```python
from build123d import *

# Parameters (mm, degrees)
SKETCH1_W                        = 6.5
SKETCH1_H                        = 60
BOSS_EXTRUDE1_DEPTH              = 6.25
CUT_EXTRUDE3_DEPTH               = 61.673820549
LPATTERN1_COUNT                  = 12
LPATTERN1_PITCH                  = 2
CBORE_FOR_M1_6_SHCS1_D           = 2.8
CBORE_FOR_M1_6_SHCS1_CBORE_D     = 5.6
CBORE_FOR_M1_6_SHCS1_CBORE_DEPTH = 1.5
SKETCH6_W                        = 1
SKETCH6_H                        = 40
CUT_EXTRUDE2_DEPTH               = 61.673820549


with BuildPart() as part:
    # Sketch1 → Boss-Extrude1 (new body)
    with BuildSketch(Plane(origin=(0, 0, 0), x_dir=(1, 0, 0), z_dir=(0, 1, 0))):
        with Locations((3.25, 30)):
            Rectangle(SKETCH1_W, SKETCH1_H)
    extrude(amount=BOSS_EXTRUDE1_DEPTH)

    # Sketch9 → Cut-Extrude3 (cut, through all)
    with BuildSketch(Plane.ZY):
        with BuildLine():
            Line((-19, 6.25), (-15, 6.25))
            Line((-15, 6.25), (-15, 5.62))
            Line((-15, 5.62), (-15.259824575, 5.62))
            ThreePointArc((-15.259824575, 5.62), (-15.358731646, 5.582771412), (-15.408543109, 5.489565217))
            ThreePointArc((-15.408543109, 5.489565217), (-15.442388286, 5.331937846), (-15.501123596, 5.181797753))
            ThreePointArc((-15.501123596, 5.181797753), (-16, 4.87), (-16.498876404, 5.181797753))
            ThreePointArc((-16.498876404, 5.181797753), (-16.557611714, 5.331937846), (-16.591456891, 5.489565217))
            ThreePointArc((-16.591456891, 5.489565217), (-16.641268354, 5.582771412), (-16.740175425, 5.62))
            Line((-16.740175425, 5.62), (-17.259824575, 5.62))
            ThreePointArc((-17.259824575, 5.62), (-17.358731646, 5.582771412), (-17.408543109, 5.489565217))
            ThreePointArc((-17.408543109, 5.489565217), (-17.442388286, 5.331937846), (-17.501123596, 5.181797753))
            ThreePointArc((-17.501123596, 5.181797753), (-18, 4.87), (-18.498876404, 5.181797753))
            ThreePointArc((-18.498876404, 5.181797753), (-18.557611714, 5.331937846), (-18.591456891, 5.489565217))
            ThreePointArc((-18.591456891, 5.489565217), (-18.641268354, 5.582771412), (-18.740175425, 5.62))
            Line((-18.740175425, 5.62), (-19, 5.62))
            Line((-19, 5.62), (-19, 6.25))
        make_face()
    cut_extrude3 = extrude(amount=-CUT_EXTRUDE3_DEPTH, mode=Mode.SUBTRACT)

    # LPattern1: Cut-Extrude3 ×12
    with Locations(*[(0, 0, -i * LPATTERN1_PITCH) for i in range(1, LPATTERN1_COUNT)]):
        add(cut_extrude3, mode=Mode.SUBTRACT)

    # CBORE for M1.6 SHCS1 (through all)
    with Locations(Plane(origin=(0, 6.25, 0), x_dir=(1, 0, 0), z_dir=(0, 1, 0))):
        with Locations((3.25, 55), (3.25, 5)):
            CounterBoreHole(CBORE_FOR_M1_6_SHCS1_D / 2, CBORE_FOR_M1_6_SHCS1_CBORE_D / 2, CBORE_FOR_M1_6_SHCS1_CBORE_DEPTH)

    # Sketch6 → Cut-Extrude2 (cut, through all)
    with BuildSketch(Plane(origin=(0, 6.25, 0), x_dir=(1, 0, 0), z_dir=(0, 1, 0))):
        with Locations((6, 20)):
            Rectangle(SKETCH6_W, SKETCH6_H)
        with Locations((0.5, 20)):
            Rectangle(SKETCH6_W, SKETCH6_H)
    extrude(amount=-CUT_EXTRUDE2_DEPTH, mode=Mode.SUBTRACT)


solid = part.part
```
Build history of the part. All positions in model axes, mm. A direction names the side the tool comes from. Round coordinates to 2 decimals unless told otherwise and drop trailing zeros. Write each loop counter-clockwise with the first axis right and the second up, starting at its lowest first coordinate (ties: lowest second). Pieces come first, ordered by that corner, then holes. Notation, with made-up numbers: (77.5, 75) -> (102.5, 75) arc R30 ccw to (102.5, 100) -> close; hole circle Ø9 at (-23.75, 24). An arc over 180 degrees is marked (long way). Put each result on its own line as item: value.
Item 1: Slice it at A-A, the plane z = -55. Give the cut face in (x, y).
Here are the results:
outline: (0, 0) -> (1.85, 0) -> (1.85, 4.75) -> (0.45, 4.75) -> (0.45, 6.25) -> (0, 6.25) -> close; (4.65, 0) -> (6.5, 0) -> (6.5, 6.25) -> (6.05, 6.25) -> (6.05, 4.75) -> (4.65, 4.75) -> close
Item 2: Wall check: probe 1 along Z at (x, y) = (3.25, 3.25); probe 2 along Z at (x, y) = (3.25, 5.7); probe 3 along X at (y, z) = (5.15, -55). Give the ranges that are in metal, low to high. Write a range as from..to.
Here are the results:
probe 1: z = -60..-56.4, -53.6..-6.4, -3.6..0
probe 2: z = -60..-57.8, -52.2..-41, -15..-7.8, -2.2..0
probe 3: x = 0..0.45, 6.05..6.5
Item 3: Slice it at D-D, the plane z = -22. Give the cut face in (x, y).
Here are the results:
outline: (1, 0) -> (5.5, 0) -> (5.5, 4.87) -> (1, 4.87) -> close
Item 4: Flat gauge pins, fed straight in: P1, Ø0.6, axis at x = 3.5, z = -27, coming from the +Y side; P2, Ø1.9, axis at y = 3, z = -15, coming from the +X side; P3, Ø2, axis at y = 3, z = -7.5, coming from the -X side. Where does each tip first touch, or does it go through?
Here are the results:
P1: stops at y = 5.62
P2: stops at x = 5.5
P3: stops at x = 1
Item 5: Slice it at C-C, the plane x = 3.25. Count the separate pieces of the cut face and the enclosed holes in it, plus the area to 3 significant figures.
Here are the results:
separate pieces: 3
enclosed holes: 0
area: 306 mm^2
Item 6: Slice it at B-B, the plane z = -5. Give the cut face in (x, y).
Here are the results:
outline: (1, 0) -> (1.85, 0) -> (1.85, 4.75) -> (1, 4.75) -> close; (4.65, 0) -> (5.5, 0) -> (5.5, 4.75) -> (4.65, 4.75) -> close
Item 7: Tool access for faces 4 (the face through (5, 4.75, -5)), 5 (the face through (3, 3, -60)): list every direction of +Z, -Z, +X, -X, +Y, -Y with a clear straight run to the whole face (end or side of a thin tool).
Here are the results:
face 4: +Y
face 5: -Z, +X, -X, +Y, -Y
Item 8: Two-plate mould, pull along Z, no slides. Class faces 1 (the face through (0.5, 2.5, -40)), 2 (the face through (3.22, 4.87, -21.99)), 3 (the face through (1, 2, -20)): pulls with the +Z half, pulls with the -Z half, needs draft (parallel to the pull), parting line crosses it, or undercut.
Here are the results:
face 1: pulls with the +Z half
face 2: undercut
face 3: needs draft
